CAD build for the part. Positions are in the model's coordinates, mm. Face numbers are marked on the shaded views. A direction names the side the tool comes from. Round coordinates to 2 decimals unless told otherwise and drop trailing zeros. Loops run counter-clockwise (first coordinate to the right, second up) from the corner with the lowest first, then second, coordinate; pieces in that order, holes last.
```python
from build123d import *

# Parameters (mm, degrees)
F0_W      = 16
F0_H      = 16
F1_DEPTH  = 5
F2_W      = 2
F2_H      = 9
F3_DEPTH  = 1.5
F4_W      = 2
F4_H      = 9
F8_W      = 0.5
F8_H      = 1
F8_H_2    = 0.5
F9_DEPTH  = 5
F10_R     = 1
F11_DEPTH = 25


# Not quite as in the source:
# - a feature names something its author has since deleted; it is built from what else it names


with BuildPart() as f1:
    # F0 (on Top) → F1 (new body)
    with BuildSketch(Plane.XY):
        with Locations((-8, 8)):
            Rectangle(F0_W, F0_H)
    extrude(amount=F1_DEPTH)

    # F2 (on face) → F3 (cut)
    with BuildSketch(Plane.XY.offset(5)):
        with Locations((-13, 11.5)):
            Rectangle(F2_W, F2_H)
        with BuildLine():
            Line((-12, 7), (-14, 7))
            ThreePointArc((-14, 7), (-8, 1), (-2, 7))
            Line((-2, 7), (-4, 7))
            ThreePointArc((-4, 7), (-8, 3), (-12, 7))
        make_face()
        with BuildLine():
            Line((-10, 16), (-12, 16))
            Line((-12, 16), (-12, 7))
            ThreePointArc((-12, 7), (-8, 3), (-4, 7))
            Line((-4, 7), (-4, 16))
            Line((-4, 16), (-6, 16))
            Line((-6, 16), (-6, 7))
            ThreePointArc((-6, 7), (-8, 5), (-10, 7))
            Line((-10, 7), (-10, 16))
        make_face()
        with Locations((-3, 11.5)):
            Rectangle(F2_W, F2_H)
    extrude(amount=-F3_DEPTH, mode=Mode.SUBTRACT)

    # F4 (on face) → F5 (revolve, cut)
    with BuildSketch(Plane.XY.offset(3.5)):
        with Locations((-13, 11.5)):
            Rectangle(F4_W, F4_H)
    revolve(axis=Axis((-12, 11.5, 3.5), (0, -1, 0)), mode=Mode.SUBTRACT)

    # F6: sweep along a path in F6_path
    with BuildLine(Plane(origin=(-10, 7, 3.5), x_dir=(0, -1, 0), z_dir=(0, 0, -1))) as f6_path:
        ThreePointArc((0, 0), (2, -2), (0, -4))
    # F5_face (on face) → F6 (sweep, cut)
    with BuildSketch(Plane(origin=(-12, 7, 2.6511736368), x_dir=(-1, 0, 0), z_dir=(0, 1, 0))):
        with BuildLine():
            Line((2, 0.8488263632), (-2, 0.8488263632))
            ThreePointArc((-2, 0.8488263632), (0, -1.1511736368), (2, 0.8488263632))
        make_face()
    sweep(path=f6_path.line, mode=Mode.SUBTRACT)

    # F4 (on face) → F7 (revolve, cut)
    with BuildSketch(Plane.XY.offset(3.5)):
        with Locations((-3, 11.5)):
            Rectangle(F4_W, F4_H)
    revolve(axis=Axis((-4, 11.5, 3.5), (0, -1, 0)), mode=Mode.SUBTRACT)

    # F8 (on face) → F9 (join)
    with BuildSketch(Plane.XY.offset(5)):
        with Locations((-13.75, 13.5)):
            Rectangle(F8_W, F8_H)
        with Locations((-10.25, 9.5)):
            Rectangle(F8_W, F8_H)
        with Locations((-5.75, 9.5)):
            Rectangle(F8_W, F8_H)
        with Locations((-2.25, 13.5)):
            Rectangle(F8_W, F8_H)
        with BuildLine():
            Line((-12.4976444751, 3.8310784478), (-12.8785175711, 3.5071406687))
            ThreePointArc((-12.8785175711, 3.5071406687), (-12.570477152, 3.1127466505), (-12.2306420128, 2.7453944767))
            Line((-12.2306420128, 2.7453944767), (-11.8497689168, 3.0693322558))
            Line((-11.8497689168, 3.0693322558), (-12.4976444751, 3.8310784478))
        make_face()
        with BuildLine():
            ThreePointArc((-3.7693579872, 2.7453944767), (-3.429522848, 3.1127466505), (-3.1214824289, 3.5071406687))
            Line((-3.1214824289, 3.5071406687), (-3.5023555249, 3.8310784478))
            Line((-3.5023555249, 3.8310784478), (-4.1502310832, 3.0693322558))
            Line((-4.1502310832, 3.0693322558), (-3.7693579872, 2.7453944767))
        make_face()
        with Locations((-8.25, 4.75)):
            Rectangle(F8_W, F8_H_2)
        with Locations((-7.75, 4.75)):
            Rectangle(F8_W, F8_H_2)
        with Locations((-8.25, 5.25)):
            Rectangle(F8_W, F8_H_2)
        with Locations((-7.75, 5.25)):
            Rectangle(F8_W, F8_H_2)
    extrude(amount=-F9_DEPTH)

    # F10 (on face) → F11 (cut)
    with BuildSketch(Plane.XY.offset(5)):
        with BuildLine():
            ThreePointArc((-7, 14), (-7.2928932188, 14.7071067812), (-8, 15))
            Line((-8, 15), (-8, 13))
            ThreePointArc((-8, 13), (-7.2928932188, 13.2928932188), (-7, 14))
        make_face()
        with BuildLine():
            Line((-8, 13), (-8, 15))
            ThreePointArc((-8, 15), (-9, 14), (-8, 13))
        make_face()
        with BuildLine():
            Line((-8, 8), (-8, 6))
            ThreePointArc((-8, 6), (-7.2928932188, 6.2928932188), (-7, 7))
            ThreePointArc((-7, 7), (-7.2928932188, 7.7071067812), (-8, 8))
        make_face()
        with BuildLine():
            ThreePointArc((-8, 8), (-9, 7), (-8, 6))
            Line((-8, 6), (-8, 8))
        make_face()
        with Locations((-14, 2)):
            Circle(F10_R)
        with Locations((-2, 2)):
            Circle(F10_R)
    extrude(amount=-F11_DEPTH, mode=Mode.SUBTRACT)


solid = f1.part
```
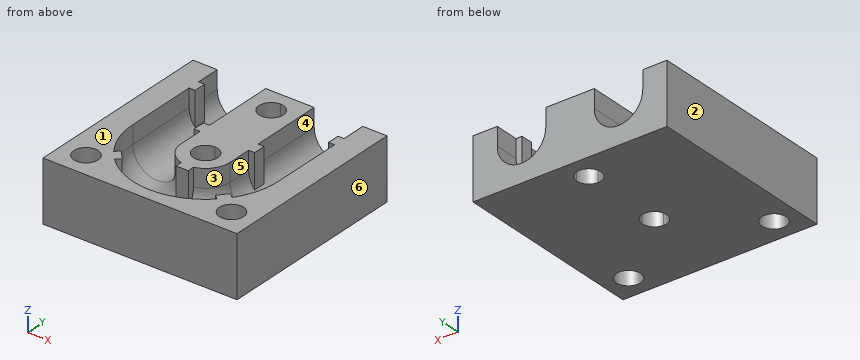
Item 1: Cut at B-B, the plane z = 3.95. State how many separate pieces and enclosed holes the cut face has, plus the area to 3 significant figures.
Answers follow:
separate pieces: 2
enclosed holes: 4
area: 125 mm2
Item 2: 3-axis set-ups, long thin cutter, end or side, ignore diameter. For the marked faces 4, 5 and 6: which of +Z, -Z, +X, -X, +Y, -Y reach the whole face in a straight line?
Answers follow:
face 4: +Z, +Y
face 5: +Z
face 6: +Z, -Z, +X, +Y, -Y
Item 3: Two-plate mould, pull along X, no slides. Class the marked faces 1, 2 and 3: released by +X, released by -X, zero draft, split by the parting line, or undercut.
Answers follow:
face 1: zero draft
face 2: released by -X
face 3: undercut
Item 4: Cut at D-D, the plane z = 0.8. Give the cut face in (x, y), plus the area to 3 significant figures.
Answers follow:
outline: (-16, 0) - (0, 0) - (0, 16) - (-16, 16) - close; hole circle Ø2 at (-14, 2); hole circle Ø2 at (-8, 7); hole circle Ø2 at (-8, 14); hole circle Ø2 at (-2, 2)
area: 243 mm2
Item 5: Cut at C-C, the plane x = -1.5. Give the cut face in (y, z).
Answers follow:
outline: (0, 0) - (1.13, 0) - (1.13, 5) - (0, 5) - close; (2.87, 0) - (16, 0) - (16, 5) - (2.87, 5) - close
Item 6: Probe line 1 (X direction, y = 10.5, z = 3.65); line 2 (X direction, y = 14.25, z = 3.9); line 3 (X direction, y = 5.75, z = 3.9). List the from-to ranges inside material, lowest first.
Answers follow:
line 1: x = -16 to -14, -10 to -6, -2 to 0
line 2: x = -16 to -14, -10 to -8.97, -7.03 to -6, -2 to 0
line 3: x = -16 to -13.87, -9.56 to -6.44, -2.13 to 0
Item 7: Flat gauge pin, fed straight in: P1, Ø5, axis at x = -2, y = 2, coming from the +Z side. Where does the tip first touch, or does it go through?
Answers follow:
P1: stops at z = 5
Item 8: Cut at A-A, the plane y = 10.25. Give the cut face in (x, z), plus the area to 3 significant figures.
Answers follow:
outline: (-16, 0) - (0, 0) - (0, 5) - (-2, 5) - (-2, 3.5) arc R2 cw to (-6, 3.5) - (-6, 5) - (-10, 5) - (-10, 3.5) arc R2 cw to (-14, 3.5) - (-14, 5) - (-16, 5) - close
area: 55.4 mm2
